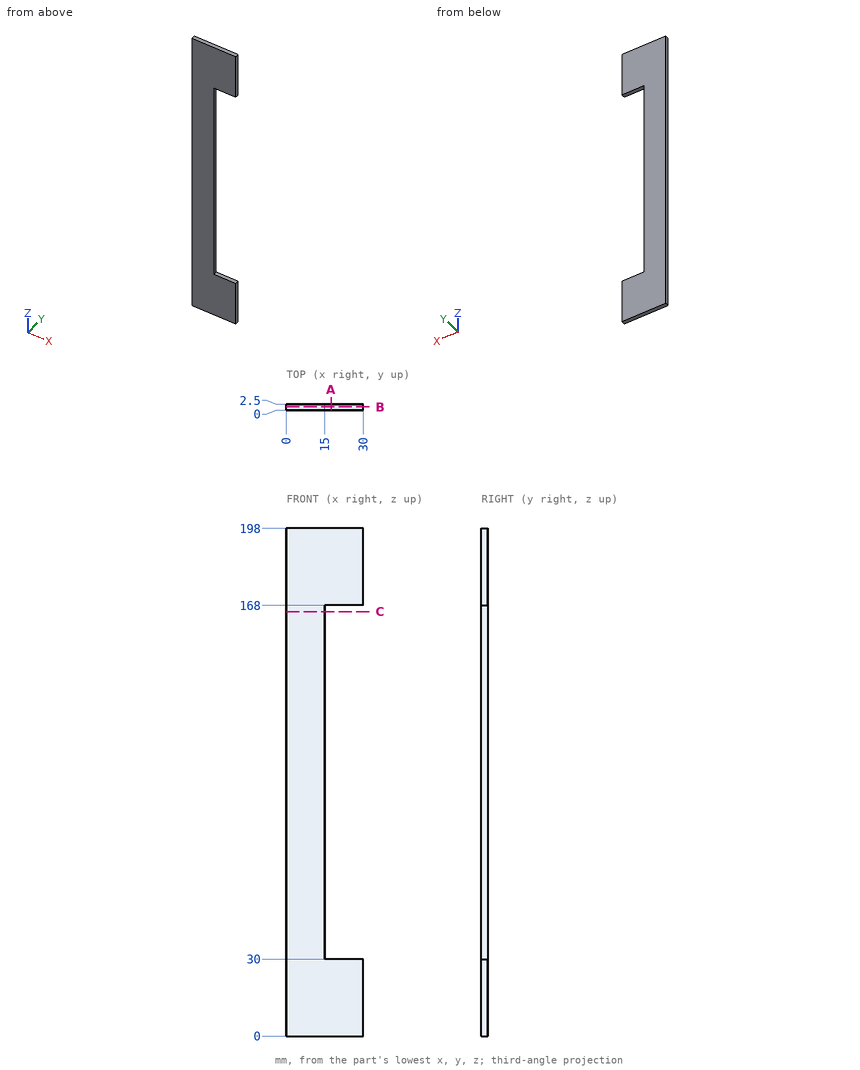
For this review, use the dimensioned drawing (mm, ordinates from the lowest corner) and the shaded views. Round coordinates to 2 decimals unless told otherwise and drop trailing zeros. Order: outer loops, then holes, each group sorted by start corner. A loop starts at its lowest first (then second) coordinate and runs counter-clockwise, first axis right, second up. Notation, with made-up numbers: M 41.5,64.25 L 99.5,64.25 A30 ccw 99.5,93.25 Z; hole C -7.5,27 d3. An arc over 180 degrees is marked long. Use a Markdown table: item, result.
1) Consider section C-C (z = 165.5). Write out the cut boundary in (x, y).
Report:
| item | result |
|---|---|
| outline | M 0,0 L 15,0 L 15,2.5 L 0,2.5 Z |
2) Consider section A-A (x = 17.5). Write out the cut boundary in (y, z), then the cut area to 3 significant figures.
Report:
| item | result |
|---|---|
| outline | M 0,0 L 2.5,0 L 2.5,30 L 0,30 Z; M 0,168 L 2.5,168 L 2.5,198 L 0,198 Z |
| area | 150 mm^2 |
3) Consider section B-B (y = 1.35). Write out the cut boundary in (x, z).
Report:
| item | result |
|---|---|
| outline | M 0,0 L 30,0 L 30,30 L 15,30 L 15,168 L 30,168 L 30,198 L 0,198 Z |
4) Insertion check: pin 1 (0.8 mm diameter, centred on y = 1, z = 114, fed in from +X). The pin has a flat end and moves straight along its axis. Give the tip position at first contact, or say it passes through.
Report:
| item | result |
|---|---|
| pin 1 | x = 15 |
5) Wall thickness on line 1 along Z through (x, y) = (18, 0.6); line 2 along X through (y, z) = (0.9, 162): over which ranges is each line inside the solid? List them lowest first. Write a range as [from, to].
Report:
| item | result |
|---|---|
| line 1 | [0, 30], [168, 198] |
| line 2 | [0, 15] |
